Design review of the part built by this model. Coordinates are the model's own, in mm. A direction names the side the tool comes from. Coordinates: 2 decimals unless noted, no trailing zeros. Order: outer loops, then holes, each group sorted by start corner. A loop starts at its lowest first (then second) coordinate and runs counter-clockwise, first axis right, second up. Notation, with made-up numbers: M 19,-3.5 L 68,-3.5 A15 cw 68,2.5 Z; hole C 86,-16 d2. An arc over 180 degrees is marked long. Answer as a JSON object with one key per item and string values.
from build123d import *

# Parameters (mm, degrees)
BOSS_EXTRUDE1_DEPTH            = 3
CUT_EXTRUDE1_REACH             = 52.648
SKETCH3_W                      = 5.5
SKETCH3_H                      = 3
BOSS_EXTRUDE2_DEPTH            = 1.5
CUT_EXTRUDE2_REACH             = 52.648
SKETCH4_W                      = 6.851042423
SKETCH4_H                      = 79.503772781
CUT_EXTRUDE2_DIRECTION_2_REACH = 52.648
BOSS_EXTRUDE3_DEPTH            = 7.5
BOSS_EXTRUDE3_DEPTH_BACK       = 7.5
BOSS_EXTRUDE5_DEPTH            = 3
CUT_EXTRUDE3_REACH             = 65.182
SKETCH10_W                     = 5.5
SKETCH10_H                     = 3
BOSS_EXTRUDE6_DEPTH            = 1.5
FILLET2_R                      = 2.75
M3_CLEARANCE_HOLE1_D           = 3.4
M3_CLEARANCE_HOLE1_CSINK_D     = 3.45
M3_CLEARANCE_HOLE1_CSINK_ANGLE = 90
M3_CLEARANCE_HOLE2_D           = 3.4
M3_CLEARANCE_HOLE2_CSINK_D     = 3.45
M3_CLEARANCE_HOLE2_CSINK_ANGLE = 90
CHAMFER2_SIZE                  = 1


with BuildPart() as part:
    # Sketch1 → Boss-Extrude1 (new body)
    with BuildSketch(Plane.XY):
        with BuildLine():
            Line((7.5, 42.5), (7.5, -42.5))
            ThreePointArc((7.5, -42.5), (0, -50), (-7.5, -42.5))
            Line((-7.5, -42.5), (-7.5, 42.5))
            ThreePointArc((-7.5, 42.5), (0, 50), (7.5, 42.5))
        make_face()
    extrude(amount=BOSS_EXTRUDE1_DEPTH)

    # Sketch2 → Cut-Extrude1 (cut, up to next)
    with BuildSketch(Plane.XY.offset(3), mode=Mode.PRIVATE) as cut_extrude1_sk1:
        with BuildLine():
            Line((-4.585044143, 42.5), (-4.585044143, 29))
            Line((-4.585044143, 29), (4.585044143, 29))
            Line((4.585044143, 29), (4.585044143, 42.5))
            ThreePointArc((4.585044143, 42.5), (0, 47.085044143), (-4.585044143, 42.5))
        make_face()
    cut_extrude1_tool1 = extrude(cut_extrude1_sk1.sketch, amount=-CUT_EXTRUDE1_REACH, mode=Mode.PRIVATE) & part.part
    cut_extrude1 = cut_extrude1_tool1.solids().sort_by_distance((0, 37.581163, 3))[0]
    add(cut_extrude1, mode=Mode.SUBTRACT)

    # Sketch3 → Boss-Extrude2 (add)
    with BuildSketch(Plane(origin=(0, 29, 0), x_dir=(1, 0, 0), z_dir=(0, 1, 0))):
        with Locations((0, -1.5)):
            Rectangle(SKETCH3_W, SKETCH3_H)
    boss_extrude2 = extrude(amount=BOSS_EXTRUDE2_DEPTH)

    # Mirror1: Cut-Extrude1, Boss-Extrude2 across plane
    add(cut_extrude1.mirror(Plane.ZX), mode=Mode.SUBTRACT)
    add(boss_extrude2.mirror(Plane.ZX))

    # Sketch4 → Cut-Extrude2 (cut, up to next)
    with BuildSketch(Plane(origin=(0, 0, 0), x_dir=(0, 0, -1), z_dir=(1, 0, 0)), mode=Mode.PRIVATE) as cut_extrude2_sk1:
        with Locations((-3.425521211, -15.751886391)):
            Rectangle(SKETCH4_W, SKETCH4_H)
    cut_extrude2_tool1 = extrude(cut_extrude2_sk1.sketch, amount=-CUT_EXTRUDE2_REACH, mode=Mode.PRIVATE) & part.part
    add(cut_extrude2_tool1.solids().sort_by_distance((0, -15.751886, 3.425521))[0], mode=Mode.SUBTRACT)

    # Sketch4 → Cut-Extrude2 direction 2 (cut, up to next)
    with BuildSketch(Plane(origin=(0, 0, 0), x_dir=(0, 0, -1), z_dir=(1, 0, 0)), mode=Mode.PRIVATE) as cut_extrude2_direction_2_sk1:
        with Locations((-3.425521211, -15.751886391)):
            Rectangle(SKETCH4_W, SKETCH4_H)
    cut_extrude2_direction_2_tool1 = extrude(cut_extrude2_direction_2_sk1.sketch, amount=CUT_EXTRUDE2_DIRECTION_2_REACH, mode=Mode.PRIVATE) & part.part
    add(cut_extrude2_direction_2_tool1.solids().sort_by_distance((0, -15.751886, 3.425521))[0], mode=Mode.SUBTRACT)

    # Sketch5 → Boss-Extrude3 (add, two sides: drawn at the far end of the back side and taken through both)
    with BuildSketch(Plane(origin=(0, 0, 0), x_dir=(0, 0, -1), z_dir=(1, 0, 0)).offset(-BOSS_EXTRUDE3_DEPTH_BACK)):
        Polygon((0, 24), (21.157354182, -34.12935287), (18.157354182, -34.12935287), (-3, 24), align=None)
    extrude(amount=BOSS_EXTRUDE3_DEPTH + BOSS_EXTRUDE3_DEPTH_BACK)

    # Sketch7 → Boss-Extrude5 (add)
    with BuildSketch(Plane.XY.offset(-21.157354182)):
        with BuildLine():
            Line((7.5, -34.12935287), (7.5, -50.62935287))
            ThreePointArc((7.5, -50.62935287), (-0.115167499, -57.896309511), (-7.5, -50.395397313))
            Line((-7.5, -50.395397313), (-7.5, -34.12935287))
            Line((-7.5, -34.12935287), (7.5, -34.12935287))
        make_face()
    extrude(amount=BOSS_EXTRUDE5_DEPTH)

    # Sketch9 → Cut-Extrude3 (cut, up to next)
    with BuildSketch(Plane(origin=(0, 0, -21.157354182), x_dir=(-1, 0, 0), z_dir=(0, 0, -1)), mode=Mode.PRIVATE) as cut_extrude3_sk1:
        with BuildLine():
            Line((-4.25, -39.12935287), (4.25, -39.12935287))
            Line((4.25, -39.12935287), (4.25, -50.395397313))
            ThreePointArc((4.25, -50.395397313), (-0.002513121, -54.647221764), (-4.25364879, -50.394020085))
            Line((-4.25364879, -50.394020085), (-4.25, -39.12935287))
        make_face()
    cut_extrude3_tool1 = extrude(cut_extrude3_sk1.sketch, amount=-CUT_EXTRUDE3_REACH, mode=Mode.PRIVATE) & part.part
    add(cut_extrude3_tool1.solids().sort_by_distance((0.001121, -46.463485, -21.157354))[0], mode=Mode.SUBTRACT)

    # Sketch10 → Boss-Extrude6 (add)
    with BuildSketch(Plane.XZ.offset(39.12935287)):
        with Locations((0, -19.657354182)):
            Rectangle(SKETCH10_W, SKETCH10_H)
    extrude(amount=BOSS_EXTRUDE6_DEPTH)

    # Fillet2
    fillet2_edges = [part.edges().sort_by_distance(p)[0] for p in [
        (2.75, -39.87935287, -18.157354182),
        (-2.75, -39.87935287, -18.157354182),
        (-2.75, 29.75, 3),
        (2.75, 29.75, 3),
    ]]
    fillet(fillet2_edges, radius=FILLET2_R - 0.0001)  # a hair under: the kernel refuses the full size

    # M3 Clearance Hole1 (through all)
    with Locations(Plane(origin=(0, 0, 0), x_dir=(-1, 0, 0), z_dir=(0, 0, -1))):
        with Locations((0, 26)):
            CounterSinkHole(M3_CLEARANCE_HOLE1_D / 2, M3_CLEARANCE_HOLE1_CSINK_D / 2, counter_sink_angle=M3_CLEARANCE_HOLE1_CSINK_ANGLE)

    # M3 Clearance Hole2 (through all)
    with Locations(Plane(origin=(0, 0, -21.157354182), x_dir=(-1, 0, 0), z_dir=(0, 0, -1))):
        with Locations((0, -36.12935287)):
            CounterSinkHole(M3_CLEARANCE_HOLE2_D / 2, M3_CLEARANCE_HOLE2_CSINK_D / 2, counter_sink_angle=M3_CLEARANCE_HOLE2_CSINK_ANGLE)

    # Chamfer2
    chamfer2_edges = [part.edges().sort_by_distance(p)[0] for p in [
        (7.5, -5.064676435, -7.578677091),
        (-7.5, -5.064676435, -7.578677091),
        (-7.5, -42.262375091, -18.157354182),
        (-0.115167499, -57.896309511, -18.157354182),
        (7.5, -42.37935287, -18.157354182),
        (0, 50, 3),
        (7.5, 33.25, 3),
        (-7.5, 33.25, 3),
    ]]
    chamfer(chamfer2_edges, length=CHAMFER2_SIZE)


solid = part.part
1) Tool access review of faces 1 (the flat face through (-5, 37, 0)), 2 (the cylindrical face through (0.101, 47.084, 1.521)), 3 (the flat face through (-7.5, -4, -10)), 4 (the cylindrical face through (-1.92, -39.89, -18.94)), 5 (the flat face through (7.5, -4, -10)): name each direction out of +Z, -Z, +X, -X, +Y, -Y from which nothing blocks a thin tool from reaching the whole face with its end or side.
Taken from the geometry:
{"face 1": "-Z, +X, -X, +Y", "face 2": "+Z, -Z", "face 3": "+Z, -Z, -X, +Y, -Y", "face 4": "+Z", "face 5": "+Z, -Z, +X, +Y, -Y"}
2) Mouldability with a two-part tool opening along Y and no side actions: class faces 6 (the flat face through (-0.11, -4.66, -10.43)), 7 (the cylindrical face through (-0.221, 27.686, 1.533)), 8 (the flat face through (4.42, -42.82, -18.157)) as released by +Y, released by -Y, zero draft, split by the parting line, or undercut.
Taken from the geometry:
{"face 6": "released by +Y", "face 7": "undercut", "face 8": "zero draft"}
3) To check wall thickness, follow L1, parallel to Z at x = 6.5, y = 28; L2, parallel to X at y = 26, z = 2.15; L3, parallel to Z at x = 6.25, y = -46.5. State the ranges of each line that lie inside material, in increasing order.
Taken from the geometry:
{"L1": "z = 0 to 3", "L2": "x = -7.35 to -1.7, 1.7 to 7.35", "L3": "z = -21.16 to -18.16"}
4) Add section B-B (z = -10.75). State the section outline as (x, y) points.
Taken from the geometry:
{"outline": "M -7.5,-10.85 L -6.5,-13.78 L 6.5,-13.78 L 7.5,-10.85 L 7.5,-5.54 L -7.5,-5.54 Z"}
5) Add section A-A (y = 33.5). State the section outline as (x, z) points, and give its area (3 significant figures).
Taken from the geometry:
{"outline": "M -7.5,0 L -4.59,0 L -4.59,3 L -6.5,3 L -7.5,2 Z; M 4.59,0 L 7.5,0 L 7.5,2 L 6.5,3 L 4.59,3 Z", "area": "16.5 mm2"}
6) Add section C-C (y = -4). State the section outline as (x, z) points, and give its area (3 significant figures).
Taken from the geometry:
{"outline": "M -7.5,-10.19 L 7.5,-10.19 L 7.5,-8.26 L 6.5,-7.19 L -6.5,-7.19 L -7.5,-8.26 Z", "area": "43.9 mm2"}
7) Insertion check: pin 1 Ø1 at (x, y) = (0, 19.5) entering from +Z; pin 2 Ø1.5 at (x, z) = (1.5, -19) entering from -Y; pin 3 Ø3.5 at (y, z) = (-42.5, -19) entering from +X; pin 4 Ø4 at (x, y) = (0.5, 16) entering from +Z. Each pin has a flat end and moves straight along its axis. Give the tip position at first contact, or say it passes through.
Taken from the geometry:
{"pin 1": "stops at z = 1.54", "pin 2": "stops at y = -57.86", "pin 3": "stops at x = 7.5", "pin 4": "stops at z = 0.82"}
